```python
from build123d import *

# Parameters (mm, degrees)
EXTRUS_O1_DEPTH               = 16
EXTRUS_O2_REACH               = 61.365
ESBO_O2_R                     = 2.55
FURO_ROSCADO_DE_M5X0_82_D     = 4.2
FURO_ROSCADO_DE_M5X0_82_DEPTH = 14
FURO_ROSCADO_DE_M5X0_82_TIP   = 1.2618073
ESBO_O5_R                     = 2.75
EXTRUS_O3_DEPTH               = 63.096698785


with BuildPart() as part:
    # Esboço1 → Extrusão1 (new body)
    with BuildSketch(Plane.XY):
        with BuildLine():
            Line((0, 0), (0, 48))
            Line((0, 48), (-8, 48))
            Line((-8, 48), (-8, 36.5))
            Line((-8, 36.5), (-44, 36.5))
            Line((-44, 36.5), (-44, 24.75))
            Line((-44, 24.75), (-34.964766161, 24.75))
            ThreePointArc((-34.964766161, 24.75), (-19, 24), (-34.964766161, 23.25))
            Line((-34.964766161, 23.25), (-44, 23.25))
            Line((-44, 23.25), (-44, 11.5))
            Line((-44, 11.5), (-8, 11.5))
            Line((-8, 11.5), (-8, 0))
            Line((-8, 0), (0, 0))
        make_face()
    extrude(amount=EXTRUS_O1_DEPTH)

    # Esboço2 → Extrusão2 (cut, up to next)
    with BuildSketch(Plane(origin=(0, 36.5, 0), x_dir=(1, 0, 0), z_dir=(0, 1, 0)), mode=Mode.PRIVATE) as extrus_o2_sk1:
        with Locations(Location((-39, -8, 0), (0, 0, 270))):
            Circle(ESBO_O2_R)
    extrus_o2_tool1 = extrude(extrus_o2_sk1.sketch, amount=-EXTRUS_O2_REACH, mode=Mode.PRIVATE) & part.part
    add(extrus_o2_tool1.solids().sort_by_distance((-39, 36.5, 8))[0], mode=Mode.SUBTRACT)

    # Furo roscado de M5x0.82
    with Locations(Plane(origin=(-39, 23.25, 8), x_dir=(1, 0, 0), z_dir=(0, 1, 0))):
        with Locations((0, 0)):
            Hole(FURO_ROSCADO_DE_M5X0_82_D / 2, depth=FURO_ROSCADO_DE_M5X0_82_DEPTH)
            with Locations((0, 0, -(FURO_ROSCADO_DE_M5X0_82_DEPTH + FURO_ROSCADO_DE_M5X0_82_TIP / 2))):  # 118° drill point
                Cone(0, FURO_ROSCADO_DE_M5X0_82_D / 2, FURO_ROSCADO_DE_M5X0_82_TIP, mode=Mode.SUBTRACT)

    # Esboço5 → Extrusão3 (cut, through all)
    with BuildSketch(Plane.ZY.offset(8)):
        with Locations(Location((8, 43, 0), (0, 0, 270))):
            Circle(ESBO_O5_R)
        with Locations(Location((8, 5, 0), (0, 0, 270))):
            Circle(ESBO_O5_R)
    extrude(amount=-EXTRUS_O3_DEPTH, mode=Mode.SUBTRACT)


solid = part.part
```
Could you check a few things on this model? Use its own coordinates, in mm. A direction names the side the tool comes from. Give positions to 0.01 mm unless a question says otherwise; leave off trailing zeros. Write each loop counter-clockwise with the first axis right and the second up, starting at its lowest first coordinate (ties: lowest second). Pieces come first, ordered by that corner, then holes. Notation, with made-up numbers: (50, 9) - (91, 9) arc R19 cw to (91, 26) - close; hole circle Ø5 at (-24.5, 1). An arc over 180 degrees is marked (long way). One line per item, written item: value. Start each with the question number.
Item 1: Imagine slicing it at B-B, the plane y = 43. List the corners of the cut face in (x, z) for me, and give its area (3 significant figures).
Item 2: If we mould it in two halves opening along Y, with no side actions, what happens to faces 4 (the face through (-17, 24, 0)), 5 (the face through (-4.06, 3.52, 10.32)), 6 (the face through (-4, 48, 8))? For each: +Y half, -Y half, draft (parallel to the pull), parting line (faces both ways), or undercut.
Item 3: Imagine slicing it at C-C, the plane z = 8. List the corners of the cut face in (x, y) for me, and give its area (3 significant figures).
Item 4: Please list where these lines run through material, in increasing order: line 1 (Z direction, x = -39, y = 17); line 2 (Z direction, x = -6.25, y = 43); line 3 (Y direction, x = -27, z = 7.75). Write a range as from..to.
Item 5: Which directions (+Z, -Z, +X, -X, +Y, -Y) give clear straight access to the entire face, cutting with the end or side of a thin tool? Please do faces 1 (the face through (-8, 8, 8)), 2 (the face through (-8, 40, 8)), 3 (the face through (-36.47, 30.71, 7.67)).
Item 6: I'm going to push flat-ended pins straight in: pin 1 (4 mm diameter, centred on x = -39, z = 8, fed in from -Y); pin 2 (4.5 mm diameter, centred on x = -37, z = 4, fed in from -Y); pin 3 (3.5 mm diameter, centred on y = 7.5, z = 11.5, fed in from -X); pin 4 (4.5 mm diameter, centred on x = -37.5, z = 11, fed in from +Y). Where does each tip first touch, or does it pass through?
Item 7: Imagine slicing it at A-A, the plane x = -27. List the corners of the cut face in (y, z) for me.
Item 8: Imagine slicing it at D-D, the plane x = -39. List the corners of the cut face in (y, z) for me, and give its area (3 significant figures).
Geometry says:
1. outline: (-8, 0) - (0, 0) - (0, 5.25) - (-8, 5.25) - close; (-8, 10.75) - (0, 10.75) - (0, 16) - (-8, 16) - close
1. area: 84.0 mm^2
2. face 4: draft
2. face 5: undercut
2. face 6: +Y half
3. outline: (-44, 11.5) - (-41.1, 11.5) - (-41.1, 23.25) - (-44, 23.25) - close; (-44, 24.75) - (-41.55, 24.75) - (-41.55, 36.5) - (-44, 36.5) - close; (-36.9, 11.5) - (-8, 11.5) - (-8, 7.75) - (0, 7.75) - (0, 40.25) - (-8, 40.25) - (-8, 36.5) - (-36.45, 36.5) - (-36.45, 24.75) - (-34.96, 24.75) arc R8 cw (long way) to (-34.96, 23.25) - (-36.9, 23.25) - close; (-8, 0) - (0, 0) - (0, 2.25) - (-8, 2.25) - close; (-8, 45.75) - (0, 45.75) - (0, 48) - (-8, 48) - close
3. area: 872 mm^2
4. line 1: 0..5.9, 10.1..16
4. line 2: 0..5.25, 10.75..16
4. line 3: 11.5..16, 32..36.5
5. face 1: +Z, -Z, -X, -Y
5. face 2: +Z, -Z, -X, +Y
5. face 3: +Y
6. pin 1: through
6. pin 2: y = 11.5
6. pin 3: x = -8
6. pin 4: y = 36.5
7. outline: (11.5, 0) - (16, 0) - (16, 16) - (11.5, 16) - close; (32, 0) - (36.5, 0) - (36.5, 16) - (32, 16) - close
8. outline: (11.5, 0) - (23.25, 0) - (23.25, 5.9) - (11.5, 5.9) - close; (11.5, 10.1) - (23.25, 10.1) - (23.25, 16) - (11.5, 16) - close; (24.75, 0) - (36.5, 0) - (36.5, 5.45) - (24.75, 5.45) - close; (24.75, 10.55) - (36.5, 10.55) - (36.5, 16) - (24.75, 16) - close
8. area: 267 mm^2
